For this review, take the finished solid that the model builds, in its own axes (mm). A direction names the side the tool comes from. Round coordinates to 2 decimals unless told otherwise and drop trailing zeros. Write each loop counter-clockwise with the first axis right and the second up, starting at its lowest first coordinate (ties: lowest second). Pieces come first, ordered by that corner, then holes. Notation, with made-up numbers: M 10.5,-20 L 43.5,-20 A29 cw 43.5,14 Z; hole C 30.25,76 d3. An arc over 180 degrees is marked long. Use one line per item in the form item = value. Start each with the question number.
Item 1: Add section B-B (z = 96). State the section outline as (x, y) points (3 decimals).
Item 2: For line 1 (X direction, y = 1.95, z = 139.7); line 2 (X direction, y = 2.2, z = 30.5) (3 decimals); line 3 (X direction, y = 1.3, z = 78) (3 decimals), list the stretches that pass through material, from the lowest coordinate up. Write a range as [from, to].
Item 3: For P1, Ø5.5, axis at x = -24.13, z = -44.958, coming from the -Y side; P2, Ø8, axis at x = -27.5, z = 45, coming from the -Y side; P3, Ø1.6, axis at x = 7, y = 2.5, coming from the +Z side; P4, Ø1, axis at x = -6, y = 1.5, coming from the -Z side, all flat-tipped, find the tip position at first contact; note any pin that passes through.
Item 4: Add section C-C (y = 2.3). Count the separate pieces of the cut face and the enclosed holes in it, and give its area (3 significant figures).
Item 5: Add section D-D (z = -94). State the section outline as (x, y) points (3 decimals).
Item 6: For faces 1 (the cylindrical face through (18.203, 1.565, -163.194)), 2 (the flat face through (21.14, 1.61, 32.81)), list the 3-axis set-ups (+Z, -Z, +X, -X, +Y, -Y) from which the entire face can be reached by the end or side of a thin tool; tool diameter is ignored.
Item 7: Add section A-A (z = 60.96). State the section outline as (x, y) points (3 decimals), and give its area (3 significant figures).
Item 8: Draft analysis for pull direction X (two halves, no side actions). For faces 3 (the flat face through (-4.803, 1.61, -4.349)), 4 (the cylindrical face through (-17.354, 1.565, 163.377)), 5 (the flat face through (5.976, 1.61, -95.057)), 6 (the flat face through (-1, 3.175, -2)), state which applies: released by +X, released by -X, zero draft, split by the parting line, or undercut.
from build123d import *

# Parameters (mm, degrees)
SKETCH1_R           = 14.478
SKETCH1_R_2         = 3.175
BOSS_EXTRUDE1_DEPTH = 3.175
CUT_EXTRUDE1_DEPTH  = 168.948797034


with BuildPart() as part:
    # Sketch1 → Boss-Extrude1 (new body)
    with BuildSketch(Plane(origin=(0, 0, 0), x_dir=(1, 0, 0), z_dir=(0, 1, 0))):
        with BuildLine():
            Line((-36.83, 65.023620999), (-36.83, -139.7))
            ThreePointArc((-36.83, -139.7), (-16.890130527, -163.46341108), (9.97478294, -147.952946058))
            Line((9.97478294, -147.952946058), (33.766385136, -82.586056251))
            ThreePointArc((33.766385136, -82.586056251), (36.058233853, -74.032760396), (36.83, -65.21143297))
            Line((36.83, -65.21143297), (36.83, 139.7))
            ThreePointArc((36.83, 139.7), (17.75430807, 163.29472123), (-9.312633231, 149.584375461))
            Line((-9.312633231, 149.584375461), (-10.51620944, 146.277577002))
            Line((-10.51620944, 146.277577002), (-33.766385136, 82.39824428))
            ThreePointArc((-33.766385136, 82.39824428), (-36.058233853, 73.844948425), (-36.83, 65.023620999))
        make_face()
        with Locations(Location((-12.7, -139.7, 0), (0, 0, 270))):
            Circle(SKETCH1_R, mode=Mode.SUBTRACT)
        with Locations(Location((-24.13, -44.958, 0), (0, 0, 270))):
            Circle(SKETCH1_R_2, mode=Mode.SUBTRACT)
        with BuildLine():
            Line((22.225, -64.262), (-22.225, -64.262))
            ThreePointArc((-22.225, -64.262), (-25.527, -60.96), (-22.225, -57.658))
            Line((-22.225, -57.658), (22.225, -57.658))
            ThreePointArc((22.225, -57.658), (25.527, -60.96), (22.225, -64.262))
        make_face(mode=Mode.SUBTRACT)
        with Locations(Location((24.242138156, -44.897632473, 0), (0, 0, 270))):
            Circle(SKETCH1_R_2, mode=Mode.SUBTRACT)
        with Locations(Location((-24.13, 44.958, 0), (0, 0, 270))):
            Circle(SKETCH1_R_2, mode=Mode.SUBTRACT)
        with BuildLine():
            ThreePointArc((-22.225, 57.658), (-25.527, 60.96), (-22.225, 64.262))
            Line((-22.225, 64.262), (22.225, 64.262))
            ThreePointArc((22.225, 64.262), (25.527, 60.96), (22.225, 57.658))
            Line((22.225, 57.658), (-22.225, 57.658))
        make_face(mode=Mode.SUBTRACT)
        with Locations(Location((24.242138156, 44.897632473, 0), (0, 0, 270))):
            Circle(SKETCH1_R_2, mode=Mode.SUBTRACT)
        with Locations(Location((12.7, 139.7, 0), (0, 0, 270))):
            Circle(SKETCH1_R, mode=Mode.SUBTRACT)
    extrude(amount=BOSS_EXTRUDE1_DEPTH)

    # Sketch2 → Cut-Extrude1 (cut, through all)
    with BuildSketch(Plane(origin=(0, 3.175, 0), x_dir=(1, 0, 0), z_dir=(0, 1, 0))):
        with BuildLine():
            Line((-27.305, 17.780518249), (-27.305, -32.670889551))
            ThreePointArc((-27.305, -32.670889551), (-24.768631727, -35.780997992), (-21.21191369, -33.922047929))
            Line((-21.21191369, -33.922047929), (12.072240801, 43.706841622))
            ThreePointArc((12.072240801, 43.706841622), (11.804914085, 46.705597944), (9.154154491, 48.133))
            Line((9.154154491, 48.133), (-12.477385793, 48.133))
            ThreePointArc((-12.477385793, 48.133), (-14.224983737, 47.608759594), (-15.395472103, 46.209158378))
            Line((-15.395472103, 46.209158378), (-27.04808631, 19.031676627))
            ThreePointArc((-27.04808631, 19.031676627), (-27.240108441, 18.419149976), (-27.305, 17.780518249))
        make_face()
        with BuildLine():
            Line((27.305, -17.780518249), (27.305, 32.670889551))
            ThreePointArc((27.305, 32.670889551), (24.768631727, 35.780997992), (21.21191369, 33.922047929))
            Line((21.21191369, 33.922047929), (-12.072240801, -43.706841622))
            ThreePointArc((-12.072240801, -43.706841622), (-11.804914085, -46.705597944), (-9.154154491, -48.133))
            Line((-9.154154491, -48.133), (12.477385793, -48.133))
            ThreePointArc((12.477385793, -48.133), (14.224983737, -47.608759594), (15.395472103, -46.209158378))
            Line((15.395472103, -46.209158378), (27.04808631, -19.031676627))
            ThreePointArc((27.04808631, -19.031676627), (27.240108441, -18.419149976), (27.305, -17.780518249))
        make_face()
        with BuildLine():
            Line((-15.725871274, -73.787), (-24.13, -73.787))
            ThreePointArc((-24.13, -73.787), (-26.37506403, -74.71693597), (-27.305, -76.962))
            Line((-27.305, -76.962), (-27.305, -100.594783353))
            ThreePointArc((-27.305, -100.594783353), (-24.669761403, -103.723566283), (-21.138522754, -101.658592024))
            Line((-21.138522754, -101.658592024), (-12.734394028, -78.025808671))
            ThreePointArc((-12.734394028, -78.025808671), (-13.131818698, -75.131285321), (-15.725871274, -73.787))
        make_face()
        with BuildLine():
            Line((-9.990759398, -118.999), (-2.24070983, -118.999))
            ThreePointArc((-2.24070983, -118.999), (-0.409995151, -118.418052576), (0.750767416, -116.887808671))
            Line((0.750767416, -116.887808671), (14.570605972, -78.025808671))
            ThreePointArc((14.570605972, -78.025808671), (14.173181302, -75.131285321), (11.579128726, -73.787))
            Line((11.579128726, -73.787), (3.829079157, -73.787))
            ThreePointArc((3.829079157, -73.787), (1.998364479, -74.367947424), (0.837601912, -75.898191329))
            Line((0.837601912, -75.898191329), (-12.982236644, -114.760191329))
            ThreePointArc((-12.982236644, -114.760191329), (-12.584811974, -117.654714679), (-9.990759398, -118.999))
        make_face()
        with BuildLine():
            Line((15.725871274, 73.787), (24.13, 73.787))
            ThreePointArc((24.13, 73.787), (26.37506403, 74.71693597), (27.305, 76.962))
            Line((27.305, 76.962), (27.305, 100.594783353))
            ThreePointArc((27.305, 100.594783353), (24.669761403, 103.723566283), (21.138522754, 101.658592024))
            Line((21.138522754, 101.658592024), (12.734394028, 78.025808671))
            ThreePointArc((12.734394028, 78.025808671), (13.131818698, 75.131285321), (15.725871274, 73.787))
        make_face()
        with BuildLine():
            Line((9.990759398, 118.999), (2.24070983, 118.999))
            ThreePointArc((2.24070983, 118.999), (0.409995151, 118.418052576), (-0.750767416, 116.887808671))
            Line((-0.750767416, 116.887808671), (-14.570605972, 78.025808671))
            ThreePointArc((-14.570605972, 78.025808671), (-14.173181302, 75.131285321), (-11.579128726, 73.787))
            Line((-11.579128726, 73.787), (-3.829079157, 73.787))
            ThreePointArc((-3.829079157, 73.787), (-1.998364479, 74.367947424), (-0.837601912, 75.898191329))
            Line((-0.837601912, 75.898191329), (12.982236644, 114.760191329))
            ThreePointArc((12.982236644, 114.760191329), (12.584811974, 117.654714679), (9.990759398, 118.999))
        make_face()
    extrude(amount=-CUT_EXTRUDE1_DEPTH, mode=Mode.SUBTRACT)


solid = part.part
Calculated:
q1.outline = M -36.83,0 L -27.305,0 L -27.305,3.175 L -36.83,3.175 Z; M -19.126,0 L -6.311,0 L -6.311,3.175 L -19.126,3.175 Z; M 8.179,0 L 28.884,0 L 28.884,3.175 L 8.179,3.175 Z
q2.line_1 = [-36.83, -27.18], [1.78, 12.98]
q2.line_2 = [-36.83, -27.305], [-19.745, -6.41], [22.131, 36.83]
q2.line_3 = [-36.83, -27.305], [-12.725, 0.09], [14.58, 35.194]
q3.P1 = through
q3.P2 = 0
q3.P3 = 154.7
q3.P4 = -155.54
q4.separate_pieces = 1
q4.enclosed_holes = 14
q4.area = 13,300 mm^2
q5.outline = M -29.544,0 L -8.89,0 L -8.89,3.175 L -29.544,3.175 Z; M 5.6,0 L 18.415,0 L 18.415,3.175 L 5.6,3.175 Z; M 27.305,0 L 36.83,0 L 36.83,3.175 L 27.305,3.175 Z
q6.face_1 = -Z, +Y, -Y
q6.face_2 = +Y, -Y
q7.outline = M -36.83,0 L -25.527,0 L -25.527,3.175 L -36.83,3.175 Z; M 25.527,0 L 36.83,0 L 36.83,3.175 L 25.527,3.175 Z
q7.area = 71.8 mm^2
q8.face_3 = undercut
q8.face_4 = split by the parting line
q8.face_5 = undercut
q8.face_6 = zero draft
